CAD build for the part. Positions are in the model's coordinates, mm. Face numbers are marked on the shaded views. Give positions to 0.01 mm unless a question says otherwise; leave off trailing zeros. Order: outer loops, then holes, each group sorted by start corner. A loop starts at its lowest first (then second) coordinate and runs counter-clockwise, first axis right, second up. Notation, with made-up numbers: M 88.25,35.5 L 139.25,35.5 A22 cw 139.25,55.5 Z; hole C -32,-30.75 d8. An arc over 180 degrees is marked long. Put each result on its own line as item: value. Start each with the question number.
1) Pin check, flat tips, straight feed: pin 1 (12 mm diameter, centred on x = 9.5, z = 22, fed in from -Y); pin 2 (10 mm diameter, centred on y = 39.5, z = 17, fed in from -X); pin 3 (15 mm diameter, centred on x = 30.5, z = 18, fed in from +Y). Stop position of each tip, or through.
2) Cut at B-B (y = 61). Write the cut outline in (x, z).
3) Drill centre lines: line 1 (X direction, y = 8.5, z = 25); line 2 (Z direction, x = 43, y = 73); line 3 (Y direction, x = 65.5, z = 6). Where is each one in solid material? Low to high. Write a range as [from, to].
4) Two-plate mould, pull along X, no slides. Class the marked faces 1, 2, 3 and 4: released by +X, released by -X, zero draft, split by the parting line, or undercut.
5) Cut at C-C (z = 29). Write the cut outline in (x, y), and give its area (3 significant figures).
6) Cut at A-A (x = 8.5). Write the cut outline in (y, z).
```python
from build123d import *

# Parameters (mm, degrees)
F0_W     = 80
F0_H     = 40
F1_DEPTH = 100
F2_T     = -3
F3_R     = 5.08
F4_R     = 5.08
F5_R     = 5.08
F6_R     = 5.08
F8_W     = 6.79958
F8_H     = 1.99898
F9_DEPTH = 20


with BuildPart() as f1:
    # F0 (on Front) → F1 (new body)
    with BuildSketch(Plane.XZ):
        with Locations((40, 20)):
            Rectangle(F0_W, F0_H)
    extrude(amount=-F1_DEPTH)

    # F2
    f2_openings = [f1.faces().sort_by_distance(p)[0] for p in [
        (40, 0, 20),
    ]]
    offset(amount=F2_T, openings=f2_openings)

    # F3
    f3_edges = [f1.edges().sort_by_distance(p)[0] for p in [
        (0, 50, 40),
    ]]
    fillet(f3_edges, radius=F3_R)

    # F4
    f4_edges = [f1.edges().sort_by_distance(p)[0] for p in [
        (80, 50, 40),
    ]]
    fillet(f4_edges, radius=F4_R)

    # F5
    f5_edges = [f1.edges().sort_by_distance(p)[0] for p in [
        (40, 100, 40),
    ]]
    fillet(f5_edges, radius=F5_R)

    # F6
    f6_edges = [f1.edges().sort_by_distance(p)[0] for p in [
        (40, 100, 0),
    ]]
    fillet(f6_edges, radius=F6_R)

    # F8 (on face) → F9 (join)
    with BuildSketch(Plane(origin=(-44.92, 44.92, 0), x_dir=(0.707107, 0.707107, 0), z_dir=(0.707107, -0.707107, 0))):
        with Locations((70.902991, 20.67943)):
            Rectangle(F8_W, F8_H)
    extrude(amount=-F9_DEPTH)


solid = f1.part
```
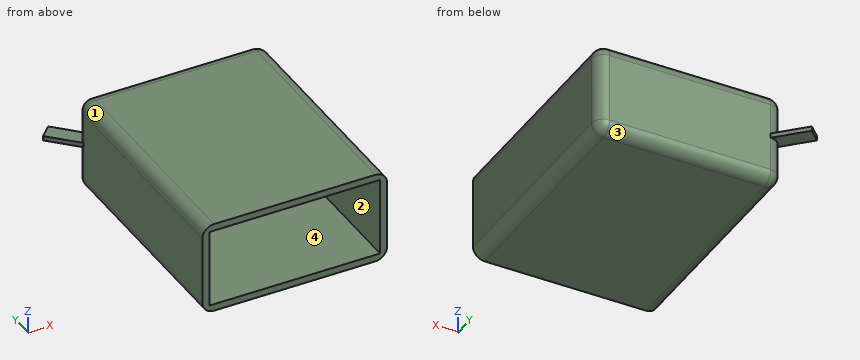
Solution:
1. pin 1: y = 93.35
1. pin 2: x = 0
1. pin 3: y = 100
2. outline: M 0,5.08 A5.08 ccw 5.08,0 L 74.92,0 A5.08 ccw 80,5.08 L 80,34.92 A5.08 ccw 74.92,40 L 5.08,40 A5.08 ccw 0,34.92 Z; hole M 3,3 L 77,3 L 77,37 L 3,37 Z
3. line 1: [0, 3], [77, 80]
3. line 2: [0, 3], [37, 40]
3. line 3: [97, 100]
4. face 1: released by -X
4. face 2: undercut
4. face 3: zero draft
4. face 4: undercut
5. outline: M 0,0 L 3,0 L 3,97 L 77,97 L 77,0 L 80,0 L 80,94.92 A5.08 ccw 74.92,100 L 5.08,100 A5.08 ccw 0,94.92 Z
5. area: 811 mm²
6. outline: M 0,0 L 94.92,0 A5.08 ccw 100,5.08 L 100,34.92 A5.08 ccw 94.92,40 L 0,40 L 0,37 L 97,37 L 97,3 L 0,3 Z
